Could you check a few things on this model? Use its own coordinates, in mm. A direction names the side the tool comes from. Coordinates: 2 decimals unless noted, no trailing zeros. Write each loop counter-clockwise with the first axis right and the second up, starting at its lowest first coordinate (ties: lowest second). Pieces come first, ordered by that corner, then holes.
```python
from build123d import *

# Parameters (mm, degrees)
SKETCH1_W           = 6
SKETCH1_H           = 6
SKETCH1_W_2         = 10
SKETCH1_H_2         = 4
SKETCH1_H_3         = 14
SKETCH1_W_3         = 34
BOSS_EXTRUDE1_DEPTH = 5
BOSS_EXTRUDE2_START = 60
SKETCH2_W           = 20
SKETCH2_H           = 28
SKETCH2_R           = 4
BOSS_EXTRUDE2_DEPTH = 60


with BuildPart() as part:
    # Sketch1 → Boss-Extrude1 (new body)
    with BuildSketch(Plane(origin=(0, 0, 0), x_dir=(0, 0, -1), z_dir=(1, 0, 0))):
        with BuildLine():
            ThreePointArc((40, 12), (42.828427125, 10.828427125), (44, 8))
            Line((44, 8), (50, 8))
            Line((50, 8), (50, 14))
            Line((50, 14), (40, 14))
            Line((40, 14), (40, 12))
        make_face()
        with BuildLine():
            Line((6, 14), (6, 8))
            Line((5.999999991, 8), (36, 8))
            ThreePointArc((36, 8), (37.171572875, 10.828427125), (40, 12))
            Line((40, 12), (40, 14))
            Line((40, 14), (6, 14))
        make_face()
        Polygon((0, 14), (0, 8), (5.999999991, 8), (6, 14), align=None)
        with Locations((-3, 11)):
            Rectangle(SKETCH1_W, SKETCH1_H)
        with BuildLine():
            ThreePointArc((-40, 12), (-37.171572875, 10.828427125), (-36, 8))
            Line((-36, 8), (-6.000000002, 8))
            Line((-6, 8), (-6, 14))
            Line((-6, 14), (-40, 14))
            Line((-40, 14), (-40, 12))
        make_face()
        with BuildLine():
            Line((-50, 14), (-50, 8))
            Line((-50, 8), (-44, 8))
            ThreePointArc((-44, 8), (-42.828427125, 10.828427125), (-40, 12))
            Line((-40, 12), (-40, 14))
            Line((-40, 14), (-50, 14))
        make_face()
        with BuildLine():
            Line((-50, 8), (-50, 4))
            Line((-50, 4), (-40, 4))
            ThreePointArc((-40, 4), (-42.828427125, 5.171572875), (-44, 8))
            Line((-44, 8), (-50, 8))
        make_face()
        with Locations((-45, 2)):
            Rectangle(SKETCH1_W_2, SKETCH1_H_2)
        with Locations((-45, -7)):
            Rectangle(SKETCH1_W_2, SKETCH1_H_3)
        with Locations((-23, -7)):
            Rectangle(SKETCH1_W_3, SKETCH1_H_3)
        with BuildLine():
            Line((-40, 4), (-40, 0))
            Line((-40, 0), (-6, 0))
            ThreePointArc((-6, 0), (-8.828427125, 1.171572875), (-10, 4))
            Line((-10, 4), (-40, 4))
        make_face()
        with BuildLine():
            ThreePointArc((-36, 8), (-37.171572875, 5.171572875), (-40, 4))
            Line((-40, 4), (-10, 4))
            ThreePointArc((-10, 4), (-8.828427126, 6.828427124), (-6.000000002, 8))
            Line((-6.000000002, 8), (-36, 8))
        make_face()
        with Locations((-3, -7)):
            Rectangle(SKETCH1_W, SKETCH1_H_3)
        with BuildLine():
            Line((0, 8), (0, 4))
            Line((0, 4), (2, 4))
            ThreePointArc((2, 4), (3.171572872, 6.828427122), (5.999999991, 8))
            Line((5.999999991, 8), (0, 8))
        make_face()
        with BuildLine():
            ThreePointArc((-6.000000002, 8), (-3.171572876, 6.828427126), (-2, 4))
            Line((-2, 4), (0, 4))
            Line((0, 4), (0, 8))
            Line((0, 8), (-6.000000002, 8))
        make_face()
        with Locations((3, -7)):
            Rectangle(SKETCH1_W, SKETCH1_H_3)
        with BuildLine():
            Line((0, 4), (0, 0))
            Line((0, 0), (6, 0))
            ThreePointArc((6, 0), (3.171572875, 1.171572875), (2, 4))
            Line((2, 4), (0, 4))
        make_face()
        with BuildLine():
            ThreePointArc((-2, 4), (-3.171572875, 1.171572875), (-6, 0))
            Line((-6, 0), (0, 0))
            Line((0, 0), (0, 4))
            Line((0, 4), (-2, 4))
        make_face()
        with BuildLine():
            ThreePointArc((10, 4), (8.828427125, 1.171572875), (6, 0))
            Line((6, 0), (40, 0))
            Line((40, 0), (40, 4))
            Line((39.999999991, 4), (10, 4))
        make_face()
        with BuildLine():
            ThreePointArc((5.999999991, 8), (8.828427122, 6.828427128), (10, 4))
            Line((10, 4), (39.999999991, 4))
            ThreePointArc((39.999999991, 4), (37.171572872, 5.171572878), (36, 8))
            Line((36, 8), (5.999999991, 8))
        make_face()
        with Locations((23, -7)):
            Rectangle(SKETCH1_W_3, SKETCH1_H_3)
        with Locations((45, -7)):
            Rectangle(SKETCH1_W_2, SKETCH1_H_3)
        with Locations((45, 2)):
            Rectangle(SKETCH1_W_2, SKETCH1_H_2)
        with BuildLine():
            ThreePointArc((44, 8), (42.828427122, 5.171572872), (39.999999991, 4))
            Line((39.999999991, 4), (50, 4))
            Line((50, 4), (50, 8))
            Line((50, 8), (44, 8))
        make_face()
    extrude(amount=BOSS_EXTRUDE1_DEPTH)

    # Sketch2 → Boss-Extrude2 (add)
    # profile 1 of 2: a face of its own
    with BuildSketch(Plane.ZY.offset(BOSS_EXTRUDE2_START)):
        with Locations((-40, 0)):
            Rectangle(SKETCH2_W, SKETCH2_H)
        with Locations((-40, 8)):
            Circle(SKETCH2_R, mode=Mode.SUBTRACT)
    # profile 2 of 2: a face of its own
    with BuildSketch(Plane.ZY.offset(BOSS_EXTRUDE2_START)):
        with Locations((40, 0)):
            Rectangle(SKETCH2_W, SKETCH2_H)
        with Locations((40, 8)):
            Circle(SKETCH2_R, mode=Mode.SUBTRACT)
    extrude(amount=-BOSS_EXTRUDE2_DEPTH)


solid = part.part
```
Item 1: If we mould it in two halves opening along Z, with no side actions, what happens to faces 1 (the flat face through (-60, 0, -40)), 2 (the flat face through (-30, 0, -30)), 3 (the flat face through (-28, 0, 50)), 4 (the flat face through (0, 0, 0))? For each: released by +Z, released by -Z, zero draft, split by the parting line, or undercut.
Item 2: Will these pins go through, and if not, where does the flat tip stop? pin 1 Ø13 at (y, z) = (8, 40) entering from -X; pin 2 Ø10 at (y, z) = (4.5, -17.5) entering from -X; pin 3 Ø12 at (x, z) = (-24, -21.5) entering from -Y.
Item 3: If I drill on line 1 along Z through (x, y) = (-15, 8); line 2 along Y through (x, z) = (-40.5, 40); line 3 along Z through (x, y) = (-11, 0.25), over which ranges is the centre line in solid material (lowest first)?
Item 4: I want a section at C-C, the plane z = 41. List the corners of the cut face in (x, y) for me.
Item 5: Which directions (+Z, -Z, +X, -X, +Y, -Y) give clear straight access to the entire face, cutting with the end or side of a thin tool? Please do faces 5 (the flat face through (-30, 0, 30)), 6 (the flat face through (-60, 0, 40)).
Item 6: I want a section at A-A, the plane x = -8. List the corners of the cut face in (y, z) for me, then the cut area to 3 significant figures.
Item 7: I want a section at D-D, the plane y = 2. List the corners of the cut face in (x, z) for me.
Item 8: I want a section at B-B, the plane y = -8. List the corners of the cut face in (x, z) for me.
Taken from the geometry:
1. face 1: zero draft
1. face 2: undercut
1. face 3: released by +Z
1. face 4: undercut
2. pin 1: stops at x = -60
2. pin 2: stops at x = 0
2. pin 3: passes through
3. line 1: z = -50 to -44, -36 to -30, 30 to 36, 44 to 50
3. line 2: y = -14 to 4, 12 to 14
3. line 3: z = -50 to -30, 30 to 50
4. outline: (-60, -14) - (5, -14) - (5, 4.13) - (-60, 4.13) - close; (-60, 11.87) - (5, 11.87) - (5, 14) - (-60, 14) - close
5. face 5: -X, +Y, -Y
5. face 6: +Z, -Z, -X, +Y, -Y
6. outline: (-14, -50) - (14, -50) - (14, -30) - (-14, -30) - close; (-14, 30) - (14, 30) - (14, 50) - (-14, 50) - close; hole circle Ø8 at (8, -40); hole circle Ø8 at (8, 40)
6. area: 1,020 mm2
7. outline: (-60, -50) - (5, -50) - (5, -9.46) - (0, -9.46) - (0, -30) - (-60, -30) - close; (-60, 30) - (0, 30) - (0, 9.46) - (5, 9.46) - (5, 50) - (-60, 50) - close; (0, -2.54) - (5, -2.54) - (5, 2.54) - (0, 2.54) - close
8. outline: (-60, -50) - (5, -50) - (5, 50) - (-60, 50) - (-60, 30) - (0, 30) - (0, -30) - (-60, -30) - close
